Model file for the job. Use its own axes, mm. A direction names the side the tool comes from. Coordinates: 2 decimals unless noted, no trailing zeros. Loops run counter-clockwise (first coordinate to the right, second up) from the corner with the lowest first, then second, coordinate; pieces in that order, holes last.
from build123d import *

# Parameters (mm, degrees)
BOSS_EXTRUDE1_DEPTH = 3


with BuildPart() as part:
    # Sketch1 → Boss-Extrude1 (new body)
    with BuildSketch(Plane(origin=(0, 0, 0), x_dir=(1, 0, 0), z_dir=(0, 1, 0))):
        Polygon((12, 65.5), (0, 65.5), (0, 59.5), (-3, 59.5), (-3, 39.5), (0, 39.5), (0, 24.5), (-3, 24.5), (-3, 4.5), (0, 4.5), (0, 0), (12, 0), (12, -3), (32, -3), (32, 0), (47, 0), (47, -3), (67, -3), (67, 0), (89, 0), (89, 4.5), (92, 4.5), (92, 24.5), (89, 24.5), (89, 39.5), (92, 39.5), (92, 59.5), (89, 59.5), (89, 65.5), (89, 68.5), (82, 68.5), (82, 65.5), (67, 65.5), (67, 68.5), (47, 68.5), (47, 65.5), (32, 65.5), (32, 68.5), (12, 68.5), align=None)
    extrude(amount=BOSS_EXTRUDE1_DEPTH)


solid = part.part
Q1. Drill centre lines: line 1 (X direction, y = 2.2, z = -1); line 2 (Z direction, x = 43.5, y = 2.15); line 3 (Z direction, x = 86, y = 2.75). Where is each one in solid material? Low to high.
Answers:
line 1: x = 0 to 89
line 2: z = -65.5 to 0
line 3: z = -68.5 to 0
Q2. Flat gauge pins, fed straight in: P1, Ø0.9, axis at y = 2, z = -67.5, coming from the +X side; P2, Ø1.5, axis at y = 1, z = -67, coming from the -X side; P3, Ø1, axis at x = 36.5, y = 1, coming from the -Z side. Where does each tip first touch, or does it go through?
Answers:
P1: stops at x = 89
P2: stops at x = 12
P3: stops at z = -65.5
Q3. Mould opens along X. For faces 1 (the flat face through (39, 1, 0)), 2 (the flat face through (90, 1, -39.5)), 3 (the flat face through (0, 1, -2)), 4 (the flat face through (32, 1, 2)) say: +X half, -X half, draft (parallel to the pull), parting line (faces both ways), or undercut.
Answers:
face 1: undercut
face 2: draft
face 3: -X half
face 4: undercut
Q4. Slice it at A-A (z = -61). List the corners of the cut face in (x, y), and give its area (3 significant figures).
Answers:
outline: (0, 0) - (89, 0) - (89, 3) - (0, 3) - close
area: 267 mm2
Q5. Which spindle directions (+Z, -Z, +X, -X, +Y, -Y) get a long thin tool onto all of the face, cutting with end or side? Do faces 5 (the flat face through (44, 3, -33)), 6 (the flat face through (12, 1, 1)), 7 (the flat face through (67, 1, 2)), 8 (the flat face through (75, 1, -65.5)), 9 (the flat face through (89, 1, -32)). Say none if no direction does.
Answers:
face 5: +Z, -Z, +X, -X, +Y
face 6: +Z, -X, +Y, -Y
face 7: +Z, +X, +Y, -Y
face 8: -Z, +Y, -Y
face 9: +X, +Y, -Y
